Build history of the part. All positions in model axes, mm. Face numbers are marked on the shaded views. A direction names the side the tool comes from. Round coordinates to 2 decimals unless told otherwise and drop trailing zeros. Write each loop counter-clockwise with the first axis right and the second up, starting at its lowest first coordinate (ties: lowest second). Pieces come first, ordered by that corner, then holes. Notation, with made-up numbers: (64.25, 77) -> (84.25, 77) arc R19 cw to (84.25, 96) -> close; hole circle Ø7 at (79.25, 25.5). An arc over 180 degrees is marked (long way). Answer in a Markdown table with one row per item.
```python
from build123d import *

# Parameters (mm, degrees)
SKETCH2_W            = 100.3
SKETCH2_H            = 98
SKETCH2_R            = 6
SKETCH2_W_2          = 56
SKETCH2_H_2          = 7.5
BOSS_EXTRUDE1_DEPTH  = 1.65
SKETCH5_W            = 39.102680246
SKETCH5_H            = 7.448129571
SKETCH5_H_2          = 8.164295876
SKETCH5_H_3          = 7.877829353
SKETCH5_H_4          = 7.304896309
BOSS_EXTRUDE4_DEPTH  = 10.2
SKETCH5_3_R          = 4.932717276
BOSS_EXTRUDE5_DEPTH  = 17.65
M3_CLEARANCE_HOLE1_D = 3.2
SKETCH6_W            = 56
SKETCH6_H            = 7.5
BOSS_EXTRUDE6_DEPTH  = 22.4
LPATTERN1_COUNT      = 4
LPATTERN1_PITCH      = 20
SKETCH5_4_W          = 19.193256971
SKETCH5_4_H          = 7.734596093
SKETCH5_4_W_2        = 12.138008325
SKETCH5_4_H_2        = 6.731963266
SKETCH5_4_W_3        = 25.352287192
SKETCH5_4_H_3        = 7.44812957
SKETCH5_4_H_4        = 5.8725637
SKETCH5_4_H_5        = 7.085146118
SKETCH5_4_H_6        = 6.875196527
SKETCH5_4_H_7        = 5.299630656
SKETCH5_4_W_4        = 9.779474484
SKETCH5_4_W_5        = 10.456028051
SKETCH5_4_W_6        = 24.003148834
SKETCH5_4_H_8        = 6.601011751
SKETCH5_4_W_7        = 10.00171886
BOSS_EXTRUDE11_DEPTH = 17.56
SKETCH5_6_W          = 17.760924361
SKETCH5_6_H          = 13.893626315
BOSS_EXTRUDE13_DEPTH = 12.7
SKETCH5_7_W          = 25.352287192
SKETCH5_7_H          = 7.734596093
BOSS_EXTRUDE14_DEPTH = 25


with BuildPart() as part:
    # Sketch2 → Boss-Extrude1 (new body)
    # profile 1 of 11: a face of its own
    with BuildSketch(Plane(origin=(0, 0, 0), x_dir=(1, 0, 0), z_dir=(0, 1, 0))):
        Rectangle(SKETCH2_W, SKETCH2_H)
        with Locations((-0.344987598, 21)):
            Circle(SKETCH2_R, mode=Mode.SUBTRACT)
        with Locations((-15.344987598, 21)):
            Circle(SKETCH2_R, mode=Mode.SUBTRACT)
        with Locations((-0.344987598, -4)):
            Circle(SKETCH2_R, mode=Mode.SUBTRACT)
        with Locations((-15.344987598, -4)):
            Circle(SKETCH2_R, mode=Mode.SUBTRACT)
        with Locations((-0.344987598, -29)):
            Circle(SKETCH2_R, mode=Mode.SUBTRACT)
        with Locations((-15.344987598, -29)):
            Circle(SKETCH2_R, mode=Mode.SUBTRACT)
        with Locations((-9.554652945, 35.059625045)):
            Rectangle(SKETCH2_W_2, SKETCH2_H_2, mode=Mode.SUBTRACT)
        with Locations((-9.554652945, 10.059625045)):
            Rectangle(SKETCH2_W_2, SKETCH2_H_2, mode=Mode.SUBTRACT)
        with Locations((-9.554652945, -14.940374955)):
            Rectangle(SKETCH2_W_2, SKETCH2_H_2, mode=Mode.SUBTRACT)
        with Locations((-9.554652945, -39.940374955)):
            Rectangle(SKETCH2_W_2, SKETCH2_H_2, mode=Mode.SUBTRACT)
    # profile 2 of 11: a face of its own
    with BuildSketch(Plane(origin=(0, 0, 0), x_dir=(1, 0, 0), z_dir=(0, 1, 0))):
        with Locations((-0.344987598, 21)):
            Circle(SKETCH2_R)
    # profile 3 of 11: a face of its own
    with BuildSketch(Plane(origin=(0, 0, 0), x_dir=(1, 0, 0), z_dir=(0, 1, 0))):
        with Locations((-15.344987598, 21)):
            Circle(SKETCH2_R)
    # profile 4 of 11: a face of its own
    with BuildSketch(Plane(origin=(0, 0, 0), x_dir=(1, 0, 0), z_dir=(0, 1, 0))):
        with Locations((-0.344987598, -4)):
            Circle(SKETCH2_R)
    # profile 5 of 11: a face of its own
    with BuildSketch(Plane(origin=(0, 0, 0), x_dir=(1, 0, 0), z_dir=(0, 1, 0))):
        with Locations((-15.344987598, -4)):
            Circle(SKETCH2_R)
    # profile 6 of 11: a face of its own
    with BuildSketch(Plane(origin=(0, 0, 0), x_dir=(1, 0, 0), z_dir=(0, 1, 0))):
        with Locations((-0.344987598, -29)):
            Circle(SKETCH2_R)
    # profile 7 of 11: a face of its own
    with BuildSketch(Plane(origin=(0, 0, 0), x_dir=(1, 0, 0), z_dir=(0, 1, 0))):
        with Locations((-15.344987598, -29)):
            Circle(SKETCH2_R)
    # profile 8 of 11: a face of its own
    with BuildSketch(Plane(origin=(0, 0, 0), x_dir=(1, 0, 0), z_dir=(0, 1, 0))):
        with Locations((-9.554652945, -39.940374955)):
            Rectangle(SKETCH2_W_2, SKETCH2_H_2)
    # profile 9 of 11: a face of its own
    with BuildSketch(Plane(origin=(0, 0, 0), x_dir=(1, 0, 0), z_dir=(0, 1, 0))):
        with Locations((-9.554652945, -14.940374955)):
            Rectangle(SKETCH2_W_2, SKETCH2_H_2)
    # profile 10 of 11: a face of its own
    with BuildSketch(Plane(origin=(0, 0, 0), x_dir=(1, 0, 0), z_dir=(0, 1, 0))):
        with Locations((-9.554652945, 10.059625045)):
            Rectangle(SKETCH2_W_2, SKETCH2_H_2)
    # profile 11 of 11: a face of its own
    with BuildSketch(Plane(origin=(0, 0, 0), x_dir=(1, 0, 0), z_dir=(0, 1, 0))):
        with Locations((-9.554652945, 35.059625045)):
            Rectangle(SKETCH2_W_2, SKETCH2_H_2)
    extrude(amount=BOSS_EXTRUDE1_DEPTH)

    # Sketch5 → Boss-Extrude4 (add)
    with BuildSketch(Plane(origin=(0, 1.65, 0), x_dir=(1, 0, 0), z_dir=(0, 1, 0))):
        with Locations((-10.643944628, 21.704739338)):
            Rectangle(SKETCH5_W, SKETCH5_H)
        with Locations((-10.643944628, 2.010165954)):
            Rectangle(SKETCH5_W, SKETCH5_H_2)
        with Locations((-10.643944628, -18.042490583)):
            Rectangle(SKETCH5_W, SKETCH5_H_3)
        with Locations((-10.643944628, -38.524846902)):
            Rectangle(SKETCH5_W, SKETCH5_H_4)
    extrude(amount=BOSS_EXTRUDE4_DEPTH)

    # Sketch5_3 → Boss-Extrude5 (add)
    with BuildSketch(Plane(origin=(0, 1.65, 0), x_dir=(1, 0, 0), z_dir=(0, 1, 0))):
        with Locations(Location((-7.9941293, 11.391944548, 0), (0, 0, 270))):
            Circle(SKETCH5_3_R)
        with BuildLine():
            ThreePointArc((-0.667240619, 7.976338656), (6.236323108, 8.047219973), (6.307204425, 14.9507837))
            ThreePointArc((6.307204425, 14.9507837), (-0.596359302, 14.879902383), (-0.667240619, 7.976338656))
        make_face()
        with Locations(Location((-7.9941293, -9.090411772, 0), (0, 0, 270))):
            Circle(SKETCH5_3_R)
        with Locations(Location((2.891598534, -9.090411772, 0), (0, 0, 270))):
            Circle(SKETCH5_3_R)
        with Locations(Location((-7.9941293, -29.143068308, 0), (0, 0, 270))):
            Circle(SKETCH5_3_R)
        with Locations(Location((2.891598534, -29.143068308, 0), (0, 0, 270))):
            Circle(SKETCH5_3_R)
    extrude(amount=BOSS_EXTRUDE5_DEPTH)

    # M3 Clearance Hole1 (through all)
    with Locations(Plane(origin=(0, 1.65, 0), x_dir=(1, 0, 0), z_dir=(0, 1, 0))):
        with Locations((46.85, -45), (46.85, 45), (-47.15, 45), (-47.15, -45)):
            Hole(M3_CLEARANCE_HOLE1_D / 2)

    # Sketch6 → Boss-Extrude6 (add)
    with BuildSketch(Plane(origin=(0, 11.85, 0), x_dir=(1, 0, 0), z_dir=(0, 1, 0))):
        with Locations((-19.092604505, 21.704739338)):
            Rectangle(SKETCH6_W, SKETCH6_H)
    boss_extrude6 = extrude(amount=BOSS_EXTRUDE6_DEPTH)

    # LPattern1: Boss-Extrude6 ×4
    with Locations(*[(0, 0, i * LPATTERN1_PITCH) for i in range(1, LPATTERN1_COUNT)]):
        add(boss_extrude6)

    # Sketch5_4 → Boss-Extrude11 (add)
    with BuildSketch(Plane(origin=(0, 1.65, 0), x_dir=(1, 0, 0), z_dir=(0, 1, 0))):
        with Locations((20.07958985, -32.007733528)):
            Rectangle(SKETCH5_4_W, SKETCH5_4_H)
        with Locations((36.756447429, -31.506417114)):
            Rectangle(SKETCH5_4_W_2, SKETCH5_4_H_2)
        with Locations((24.44820431, -23.270504608)):
            Rectangle(SKETCH5_4_W_3, SKETCH5_4_H_3)
        with Locations((20.07958985, -11.955076991)):
            Rectangle(SKETCH5_4_W, SKETCH5_4_H_3)
        with Locations((36.756447429, -11.167294056)):
            Rectangle(SKETCH5_4_W_2, SKETCH5_4_H_4)
        with Locations((24.44820431, -3.542573059)):
            Rectangle(SKETCH5_4_W_3, SKETCH5_4_H_5)
        with Locations((20.07958985, 7.954346285)):
            Rectangle(SKETCH5_4_W, SKETCH5_4_H_6)
        with Locations((36.756447429, 8.74212922)):
            Rectangle(SKETCH5_4_W_2, SKETCH5_4_H_7)
        with Locations((20.07958985, 28.794785756)):
            Rectangle(SKETCH5_4_W, SKETCH5_4_H_2)
        with Locations((36.756447429, 28.794785756)):
            Rectangle(SKETCH5_4_W_2, SKETCH5_4_H_2)
        with Locations((42.014085148, -3.542573059)):
            Rectangle(SKETCH5_4_W_4, SKETCH5_4_H_5)
        with Locations((42.352361931, -23.270504608)):
            Rectangle(SKETCH5_4_W_5, SKETCH5_4_H_3)
        with Locations((24.900529113, 17.0913323)):
            Rectangle(SKETCH5_4_W_6, SKETCH5_4_H_8)
        Polygon((28.243885726, 33.87956652), (28.243885726, 32.160767389), (29.676218336, 32.160767389), (30.687443267, 32.160767389), (42.825451592, 32.160767389), (47.580375957, 32.160767389), (47.580375957, 40.038596742), (28.243885726, 40.038596742), align=None)
        with Locations((41.90296296, 17.0913323)):
            Rectangle(SKETCH5_4_W_7, SKETCH5_4_H_8)
        with Locations((24.44820431, -43.323161144)):
            Rectangle(SKETCH5_4_W_3, SKETCH5_4_H_3)
    extrude(amount=BOSS_EXTRUDE11_DEPTH)

    # Sketch5_6 → Boss-Extrude13 (add)
    with BuildSketch(Plane(origin=(0, 1.65, 0), x_dir=(1, 0, 0), z_dir=(0, 1, 0))):
        with Locations((19.363423546, 40.826379678)):
            Rectangle(SKETCH5_6_W, SKETCH5_6_H)
    extrude(amount=BOSS_EXTRUDE13_DEPTH)

    # Sketch5_7 → Boss-Extrude14 (add)
    with BuildSketch(Plane(origin=(0, 1.65, 0), x_dir=(1, 0, 0), z_dir=(0, 1, 0))):
        with Locations((-19.524406809, 37.746864567)):
            Rectangle(SKETCH5_7_W, SKETCH5_7_H)
    extrude(amount=BOSS_EXTRUDE14_DEPTH)


solid = part.part
```
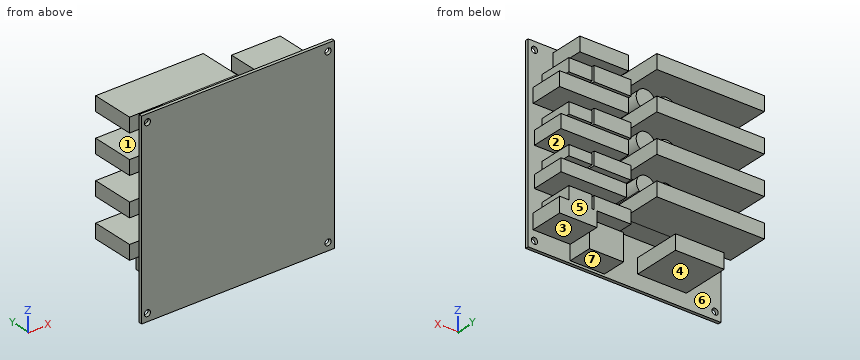
Q1. Saw through at A-A on z = 45. Write the cut outline in (x, y), plus the area to 3 significant figures.
A:
| item | result |
|---|---|
| outline | (-50.15, 0) -> (-48.75, 0) -> (-48.75, 1.65) -> (-50.15, 1.65) -> close; (-45.55, 0) -> (45.25, 0) -> (45.25, 1.65) -> (37.12, 1.65) -> (37.12, 19.21) -> (11.77, 19.21) -> (11.77, 1.65) -> (-45.55, 1.65) -> close; (48.45, 0) -> (50.15, 0) -> (50.15, 1.65) -> (48.45, 1.65) -> close |
| area | 600 mm² |
Q2. Saw through at B-B on z = -38. Write the cut outline in (x, y), plus the area to 3 significant figures.
A:
| item | result |
|---|---|
| outline | (-50.15, 0) -> (50.15, 0) -> (50.15, 1.65) -> (47.58, 1.65) -> (47.58, 19.21) -> (28.24, 19.21) -> (28.24, 14.35) -> (10.48, 14.35) -> (10.48, 1.65) -> (-6.85, 1.65) -> (-6.85, 26.65) -> (-32.2, 26.65) -> (-32.2, 1.65) -> (-50.15, 1.65) -> close |
| area | 1,360 mm² |
Q3. Two-plate mould, pull along Z, no slides. Class the marked faces 5, 6 and 7: released by +Z, released by -Z, zero draft, split by the parting line, or undercut.
A:
| item | result |
|---|---|
| face 5 | zero draft |
| face 6 | undercut |
| face 7 | released by -Z |
Q4. Wall check: line 1 (X direction, y = 13, z = 29); line 2 (Z direction, x = 46.85, y = 0.7); line 3 (X direction, y = 1.05, z = 45). Give the ranges that are in metal, low to high. Write a range as [from, to].
A:
| item | result |
|---|---|
| line 1 | [-12.92, -3.06], [-2.04, 7.82], [10.48, 29.68], [30.69, 42.83] |
| line 2 | [-49, -46.6], [-43.4, 43.4], [46.6, 49] |
| line 3 | [-50.15, -48.75], [-45.55, 45.25], [48.45, 50.15] |
Q5. Drop flat-ended pins along their axis: P1, Ø6, axis at y = 10.5, z = 22.5, coming from the +X side; P2, Ø5, axis at x = 25.5, y = 5.5, coming from the -Z side; P3, Ø6.5, axis at x = -26, y = 21, coming from the -Z side. Give the stop position or say it passes through.
A:
| item | result |
|---|---|
| P1 | x = 47.58 |
| P2 | z = -47.77 |
| P3 | z = -41.61 |
Q6. Which spindle directions (+Z, -Z, +X, -X, +Y, -Y) get a long thin tool onto all of the face, cutting with end or side? Do the marked faces 1, 2, 3 and 4. Say none if no direction does.
A:
| item | result |
|---|---|
| face 1 | -X, +Y |
| face 2 | +X, +Y |
| face 3 | -Z, +X, +Y |
| face 4 | -Z, -X, +Y |
